The drawing under review shows one solid part. Ordinate dimensions are in mm from its lowest x, y, z. A direction names the side the tool comes from. Give positions to 0.01 mm unless a question says otherwise; leave off trailing zeros. Write each loop counter-clockwise with the first axis right and the second up, starting at its lowest first coordinate (ties: lowest second). Pieces come first, ordered by that corner, then holes. Notation, with made-up numbers: M 83.25,-12 L 88.25,-12 A10 cw 88.25,7 Z; hole C -33.75,-28.75 d2. An arc over 180 degrees is marked long. Write each question's results on one line, items separated by ' | '. Start each with the question number.
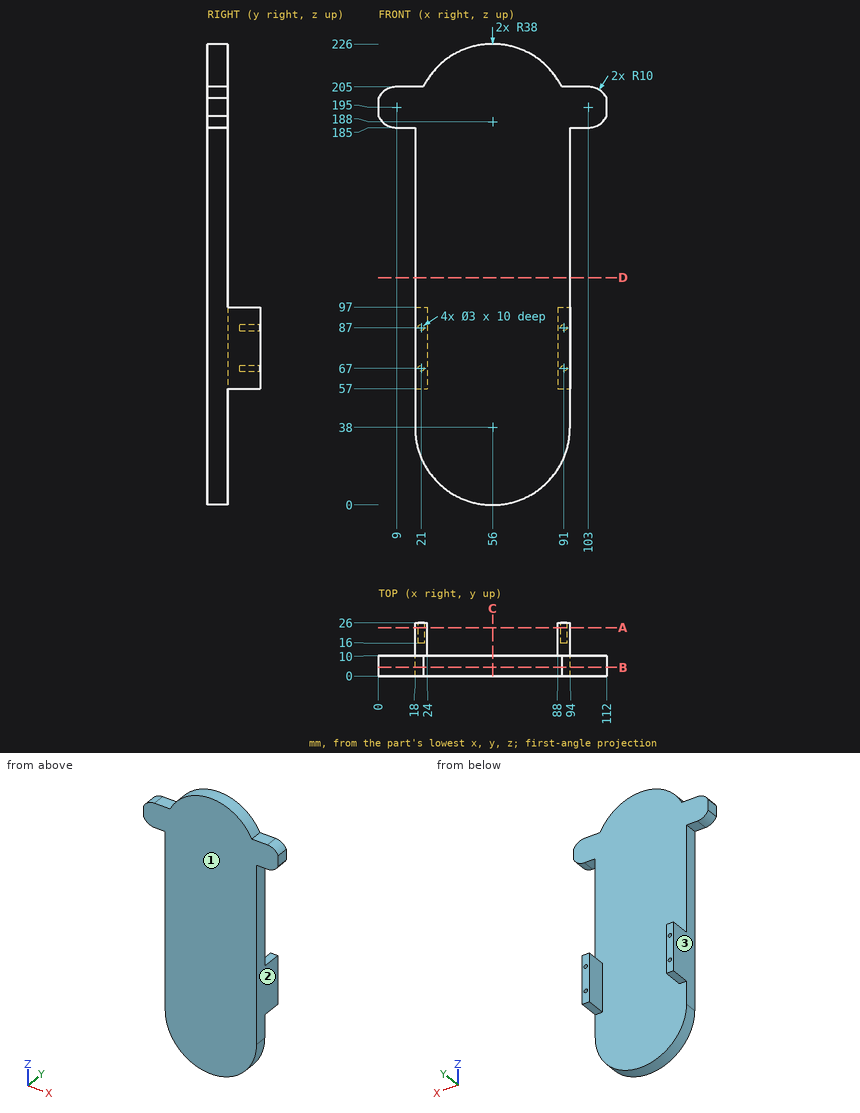
Q1. We need section D-D on z = 111.5. Write out the cut boundary in (x, y).
Q2. We need section C-C on x = 56. Write out the cut boundary in (y, z), and give its area (3 significant figures).
Q3. Wall thickness on line 1 along Z through (x, y) = (91, 19.5); line 2 along X through (y, z) = (20, 87); line 3 along Y through (x, z) = (37, 43.5): over which ranges is each line inside the solid? List them lowest first. Write a range as from..to.
Q4. We need section A-A on y = 23.75. Write out the cut boundary in (x, z), and give its area (3 significant figures).
Q5. For pin 1 Ø3 at (y, z) = (4.5, 55) entering from -X; pin 2 Ø7 at (x, y) = (99.5, 4.5) entering from -Z; pin 3 Ø2 at (x, z) = (60.5, 67) entering from +Y, all flat-tipped, find the tip position at first contact; note any pin that passes through.
Q6. We need section B-B on y = 4.25. Write out the cut boundary in (x, z).
Q7. For the marked faces 1, 2 and 3, list the 3-axis set-ups (+Z, -Z, +X, -X, +Y, -Y) from which the entire face can be reached by the end or side of a thin tool; tool diameter is ignored.
Answer sheet:
1) outline: M 18,0 L 94,0 L 94,10 L 18,10 Z
2) outline: M 0,0 L 10,0 L 10,226 L 0,226 Z | area: 2,260 mm^2
3) line 1: 57..65.5, 68.5..85.5, 88.5..97 | line 2: 18..19.5, 22.5..24, 88..89.5, 92.5..94 | line 3: 0..10
4) outline: M 18,57 L 24,57 L 24,97 L 18,97 Z; M 88,57 L 94,57 L 94,97 L 88,97 Z; hole C 21,67 d3; hole C 21,87 d3; hole C 91,67 d3; hole C 91,87 d3 | area: 452 mm^2
5) pin 1: x = 18 | pin 2: z = 185 | pin 3: y = 10
6) outline: M 0,190.64 A10 ccw 9,185 L 18,185 L 18,38 A38 ccw 94,38 L 94,185 L 103,185 A10 ccw 112,190.64 L 112,199.36 A10 ccw 103,205 L 89.99,205 A38 ccw 22.01,205 L 9,205 A10 ccw 0,199.36 Z
7) face 1: +Z, -Z, +X, -X, -Y | face 2: -Z, +X, +Y, -Y | face 3: -Z, -X, +Y, -Y
